CAD build for the part. Positions are in the model's coordinates, mm. A direction names the side the tool comes from. Give positions to 0.01 mm unless a question says otherwise; leave off trailing zeros. Loops run counter-clockwise (first coordinate to the right, second up) from the corner with the lowest first, then second, coordinate; pieces in that order, holes last. Notation, with made-up numbers: (85.25, -39) -> (117.25, -39) arc R11 ccw to (117.25, -24) -> close; hole circle Ø2 at (24, 51). An arc over 180 degrees is marked (long way). Use one line per item in the form item = value.
```python
from build123d import *

# Parameters (mm, degrees)
F1_DEPTH = 76.2
F3_DEPTH = 25.4
F5_D     = 8.73125
F7_D     = 5.1054
F8_R     = 3.175


with BuildPart() as f1:
    # F0 (on Right) → F1 (new body, symmetric)
    with BuildSketch(Plane.YZ):
        Polygon((6.3499999233, 203.2), (0, 203.2), (0, 0), (76.2, 0), (76.2, 6.3499999233), (6.3499999233, 6.3499999233), align=None)
    extrude(amount=F1_DEPTH, both=True)

    # F2 (on face) → F3 (cut)
    with BuildSketch(Plane.XZ):
        with BuildLine():
            ThreePointArc((-40.878125, 158.75), (-47.625, 165.496875), (-54.371875, 158.75))
            Line((-54.371875, 158.75), (-54.371875, 107.95))
            ThreePointArc((-54.371875, 107.95), (-47.625, 101.203125), (-40.878125, 107.95))
            Line((-40.878125, 107.95), (-40.878125, 158.75))
        make_face()
        with BuildLine():
            Line((54.371875, 107.95), (54.371875, 158.75))
            ThreePointArc((54.371875, 158.75), (47.625, 165.496875), (40.878125, 158.75))
            Line((40.878125, 158.75), (40.878125, 107.95))
            ThreePointArc((40.878125, 107.95), (47.625, 101.203125), (54.371875, 107.95))
        make_face()
    extrude(amount=-F3_DEPTH, mode=Mode.SUBTRACT)

    # F5 (through all)
    with Locations(Plane.XY.offset(6.3499999233)):
        with Locations((-44.45, 38.1), (44.45, 38.1)):
            Hole(F5_D / 2)

    # F7 (through all)
    with Locations(Plane.XY.offset(6.3499999233)):
        with Locations((15.875, 38.1), (-15.875, 38.1)):
            Hole(F7_D / 2)

    # F8
    f8_edges = [f1.edges().sort_by_distance(p)[0] for p in [
        (0, 6.35, 6.35),
        (0, 6.35, 203.2),
        (0, 76.2, 6.35),
    ]]
    fillet(f8_edges, radius=F8_R)


solid = f1.part
```
1. Drop flat-ended pins along their axis: P1, Ø8, axis at x = 15.5, z = 65.5, coming from the +Y side; P2, Ø3, axis at y = 8.5, z = 100, coming from the -X side; P3, Ø10, axis at x = 44.45, y = 38.1, coming from the +Z side. Give the stop position or say it passes through.
Result sheet:
P1 = 6.35
P2 = through
P3 = 6.35
2. Cut at D-D, the plane y = 51. Write the cut outline in (x, z), then the cut area to 3 significant figures.
Result sheet:
outline = (-76.2, 0) -> (76.2, 0) -> (76.2, 6.35) -> (-76.2, 6.35) -> close
area = 968 mm^2
3. Drill centre lines: line 1 (X direction, y = 38, z = 3); line 2 (Y direction, x = 44.45, z = 3.75); line 3 (Z direction, x = 9, y = 34.5). Where is each one in solid material? Low to high.
Result sheet:
line_1 = -76.2 to -48.81, -40.09 to -18.43, -13.32 to 13.32, 18.43 to 40.09, 48.81 to 76.2
line_2 = 0 to 33.73, 42.47 to 76.15
line_3 = 0 to 6.35
4. Tool access for faces 1 (the flat face through (1, 6.35, 103)), 2 (the cylindrical face through (-15.32, 35.61, 3.13)), 3 (the cylindrical face through (-47.773, 3.131, 101.205)): list every direction of +Z, -Z, +X, -X, +Y, -Y with a clear straight run to the whole face (end or side of a thin tool).
Result sheet:
face_1 = +Z, +X, -X, +Y
face_2 = +Z, -Z
face_3 = +Y, -Y
5. Cut at B-B, the plane x = -45.5. State how many separate pieces and enclosed holes the cut face has, then the cut area to 3 significant figures.
Result sheet:
separate_pieces = 3
enclosed_holes = 0
area = 1,270 mm^2
6. Cut at C-C, the plane x = 1. Write the cut outline in (y, z) (3 decimals), then the cut area to 3 significant figures.
Result sheet:
outline = (0, 0) -> (76.2, 0) -> (76.2, 3.175) arc R3.175 ccw to (73.025, 6.35) -> (9.525, 6.35) arc R3.175 cw to (6.35, 9.525) -> (6.35, 200.025) arc R3.175 ccw to (3.175, 203.2) -> (0, 203.2) -> close
area = 1,730 mm^2
7. Cut at A-A, the plane y = 38.1. Write the cut outline in (x, z).
Result sheet:
outline = (-76.2, 0) -> (-48.82, 0) -> (-48.82, 6.35) -> (-76.2, 6.35) -> close; (-40.08, 0) -> (-18.43, 0) -> (-18.43, 6.35) -> (-40.08, 6.35) -> close; (-13.32, 0) -> (13.32, 0) -> (13.32, 6.35) -> (-13.32, 6.35) -> close; (18.43, 0) -> (40.08, 0) -> (40.08, 6.35) -> (18.43, 6.35) -> close; (48.82, 0) -> (76.2, 0) -> (76.2, 6.35) -> (48.82, 6.35) -> close
8. Mould opens along Y. For faces 4 (the cylindrical face through (16.4, 35.6, 3.1)), 5 (the flat face through (1, 0, 103)), 6 (the flat face through (-76.2, 4, 72)) say: pulls with the +Y half, pulls with the -Y half, needs draft (parallel to the pull), parting line crosses it, or undercut.
Result sheet:
face_4 = undercut
face_5 = pulls with the -Y half
face_6 = needs draft
